```python
from build123d import *

# Parameters (mm, degrees)
F0_W     = 1219.2
F0_H     = 406.4
F1_DEPTH = 6.35
F2_W     = 101.6
F2_H     = 101.6
F3_DEPTH = 457.2


with BuildPart() as f1:
    # F0 (on Top) → F1 (new body)
    with BuildSketch(Plane.XY):
        Polygon((812.8, 148.752724), (609.6, -203.2), (1005.546815, -431.8), (1208.746815, -79.847276), align=None)
        Polygon((812.8, 148.752724), (609.6, 203.2), (609.6, -203.2), align=None)
        Rectangle(F0_W, F0_H)
        Polygon((-609.6, -203.2), (-609.6, 203.2), (-812.8, 148.752724), align=None)
        Polygon((-1005.546815, -431.8), (-609.6, -203.2), (-812.8, 148.752724), (-1208.746815, -79.847276), align=None)
    extrude(amount=F1_DEPTH)

    # F2 (on face) → F3 (join)
    with BuildSketch(Plane(origin=(0, 0, 0), x_dir=(1, 0, 0), z_dir=(0, 0, -1))):
        Polygon((-968.358634, 293.011819), (-917.558634, 381), (-1005.546815, 431.8), (-1056.346815, 343.811819), align=None)
        Polygon((-1208.746815, 79.847276), (-1120.758634, 29.047276), (-1069.958634, 117.035457), (-1157.946815, 167.835457), align=None)
        Polygon((-900.788181, -97.952724), (-812.8, -148.752724), (-762, -60.764543), (-849.988181, -9.964543), align=None)
        with Locations((-558.8, -152.4)):
            Rectangle(F2_W, F2_H)
        Polygon((968.358634, 293.011819), (1056.346815, 343.811819), (1005.546815, 431.8), (917.558634, 381), align=None)
        Polygon((1120.758634, 29.047276), (1208.746815, 79.847276), (1157.946815, 167.835457), (1069.958634, 117.035457), align=None)
        Polygon((812.8, -148.752724), (900.788181, -97.952724), (849.988181, -9.964543), (762, -60.764543), align=None)
        with Locations((558.8, -152.4)):
            Rectangle(F2_W, F2_H)
    extrude(amount=F3_DEPTH)


solid = f1.part
```
Build history of the part. All positions in model axes, mm. A direction names the side the tool comes from. Round coordinates to 2 decimals unless told otherwise and drop trailing zeros. Write each loop counter-clockwise with the first axis right and the second up, starting at its lowest first coordinate (ties: lowest second). Pieces come first, ordered by that corner, then holes.
1) Drill centre lines: probe 1 along X at (y, z) = (111, -355.5); probe 2 along Z at (x, y) = (425, -99.5); probe 3 along X at (y, z) = (-342, -233.5). Where is each one in solid material? Low to high.
2) Band-saw the part on D-D, the plane x = -633. List the corners of the cut face in (y, z), and give its area (3 significant figures).
3) Band-saw the part on C-C, the plane x = 209. List the corners of the cut face in (y, z), and give its area (3 significant figures).
4) 3-axis set-ups, long thin cutter, end or side, ignore diameter. For faces 5 (the flat face through (-508, 153, -225)), 6 (the flat face through (-1095.71, -72.43, -225.4)), 7 (the flat face through (1138, -99, -457.2)), 8 (the flat face through (1114.57, -142.79, -225.4)): which of +Z, -Z, +X, -X, +Y, -Y reach the whole face in a straight line?
5) Mould opens along X. For faces 1 (the flat face through (1011.74, -318.06, -225.4)), 2 (the flat face through (-560, 152, -457.2)), 3 (the flat face through (-1173.458, -140.97, -222.18)), 4 (the flat face through (-16, -20, 0)) say: +X half, -X half, draft (parallel to the pull), parting line (faces both ways), or undercut.
6) Pin check, flat tips, straight feed: pin 1 (10 mm diameter, centred on y = -70.5, z = -261.5, fed in from -X); pin 2 (4 mm diameter, centred on x = 806.5, z = -146.5, fed in from -Y); pin 3 (1 mm diameter, centred on x = -794, z = -183.5, fed in from -Y). Stop position of each tip, or through.
7) Band-saw the part on A-A, the plane z = -216. Give the number of separate pieces and of enclosed holes in the cut face, and give its area (3 significant figures).
8) Band-saw the part on B-B, the plane y = -319. List the corners of the cut face in (x, z), and give its area (3 significant figures).
Ans:
1. probe 1: x = -878.19 to -791, -609.6 to -508, 508 to 609.6, 791 to 878.19
1. probe 2: z = 0 to 6.35
1. probe 3: x = -1053.21 to -940.08, 940.08 to 1053.21
2. outline: (-216.71, 0) - (196.93, 0) - (196.93, 6.35) - (-216.71, 6.35) - close
2. area: 2,630 mm2
3. outline: (-203.2, 0) - (203.2, 0) - (203.2, 6.35) - (-203.2, 6.35) - close
3. area: 2,580 mm2
4. face 5: -Z, +Y, -Y
4. face 6: -Z, +Y
4. face 7: -Z, +X, -X, +Y, -Y
4. face 8: -Z, -Y
5. face 1: +X half
5. face 2: draft
5. face 3: -X half
5. face 4: undercut
6. pin 1: stops at x = -1201.22
6. pin 2: stops at y = 33.92
6. pin 3: stops at y = 42
7. separate pieces: 8
7. enclosed holes: 0
7. area: 82,600 mm2
8. outline: (-1070.67, 0) - (-1013.37, 0) - (-1013.37, -457.2) - (-953.35, -457.2) - (-953.35, 0) - (-810.17, 0) - (-810.17, 6.35) - (-1070.67, 6.35) - close; (810.17, 0) - (953.35, 0) - (953.35, -457.2) - (1013.37, -457.2) - (1013.37, 0) - (1070.67, 0) - (1070.67, 6.35) - (810.17, 6.35) - close
8. area: 58,200 mm2
